Model file for the job. Use its own axes, mm. Coordinates: 2 decimals unless noted, no trailing zeros. Loops run counter-clockwise (first coordinate to the right, second up) from the corner with the lowest first, then second, coordinate; pieces in that order, holes last. Notation, with made-up numbers: (23, -25.75) - (42, -25.75) arc R24 ccw to (42, -0.75) - close; hole circle Ø8 at (46, -35.5). An arc over 180 degrees is marked (long way). Write each question's results on one line, items separated by ' | '. Start each with the question number.
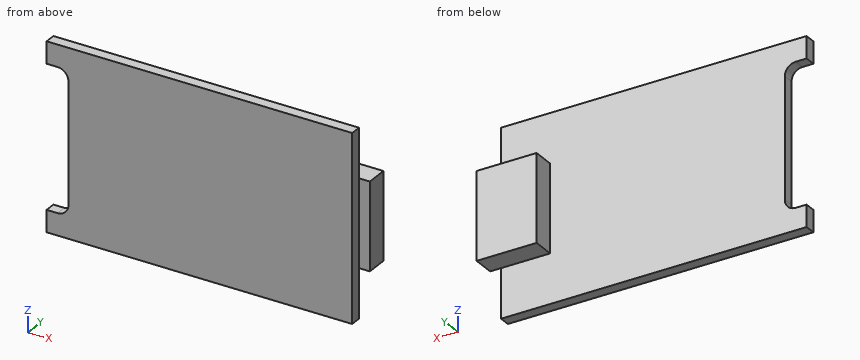
```python
from build123d import *

# Parameters (mm, degrees)
SKETCH1_W           = 28
SKETCH1_H           = 17
BOSS_EXTRUDE1_DEPTH = 1
SKETCH2_W           = 5.5
SKETCH2_H           = 8
BOSS_EXTRUDE2_DEPTH = 2
SKETCH3_W           = 2
SKETCH3_H           = 13
CUT_EXTRUDE1_DEPTH  = 18.356554958
FILLET1_R           = 1


with BuildPart() as part:
    # Sketch1 → Boss-Extrude1 (new body)
    with BuildSketch(Plane(origin=(0, 0, 0), x_dir=(1, 0, 0), z_dir=(0, 1, 0))):
        Rectangle(SKETCH1_W, SKETCH1_H)
    extrude(amount=BOSS_EXTRUDE1_DEPTH)

    # Sketch2 → Boss-Extrude2 (add)
    with BuildSketch(Plane(origin=(0, 1, 0), x_dir=(1, 0, 0), z_dir=(0, 1, 0))):
        with Locations((12.25, 0)):
            Rectangle(SKETCH2_W, SKETCH2_H)
    extrude(amount=BOSS_EXTRUDE2_DEPTH)

    # Sketch3 → Cut-Extrude1 (cut, through all)
    with BuildSketch(Plane(origin=(0, 1, 0), x_dir=(1, 0, 0), z_dir=(0, 1, 0))):
        with Locations((-13, 0)):
            Rectangle(SKETCH3_W, SKETCH3_H)
    extrude(amount=-CUT_EXTRUDE1_DEPTH, mode=Mode.SUBTRACT)

    # Fillet1
    fillet1_edges = [part.edges().sort_by_distance(p)[0] for p in [
        (-12, 0.5, -6.5),
        (-12, 0.5, 6.5),
    ]]
    fillet(fillet1_edges, radius=FILLET1_R)


solid = part.part
```
Q1. Cut at D-D (z = -4.75). List the corners of the cut face in (x, y), and give its area (3 significant figures).
Q2. Pin check, flat tips, straight feed: pin 1 (0.8 mm diameter, centred on x = 14.5, z = -1, fed in from -Y); pin 2 (0.6 mm diameter, centred on x = 12.5, y = 2, fed in from +Z); pin 3 (1.6 mm diameter, centred on y = 2, z = 1.5, fed in from -X). Stop position of each tip, or through.
Q3. Cut at B-B (x = 13). List the corners of the cut face in (y, z), and give its area (3 significant figures).
Q4. Cut at A-A (z = 1). List the corners of the cut face in (x, y), and give its area (3 significant figures).
Q5. Cut at C-C (y = 2.1). List the corners of the cut face in (x, z), and give its area (3 significant figures).
Q6. Drill centre lines: L1, parallel to Y at x = 6.25, z = 6.75; L2, parallel to Z at x = 11, y = 1.35; L3, parallel to X at y = 2.7, z = -3.75. Where is each one in solid material? Low to high. Write a range as from..to.
Check result:
1) outline: (-12, 0) - (14, 0) - (14, 1) - (-12, 1) - close | area: 26.0 mm²
2) pin 1: y = 1 | pin 2: z = 4 | pin 3: x = 9.5
3) outline: (0, -8.5) - (1, -8.5) - (1, -4) - (3, -4) - (3, 4) - (1, 4) - (1, 8.5) - (0, 8.5) - close | area: 33.0 mm²
4) outline: (-12, 0) - (14, 0) - (14, 1) - (15, 1) - (15, 3) - (9.5, 3) - (9.5, 1) - (-12, 1) - close | area: 37.0 mm²
5) outline: (9.5, -4) - (15, -4) - (15, 4) - (9.5, 4) - close | area: 44.0 mm²
6) L1: 0..1 | L2: -4..4 | L3: 9.5..15
